from build123d import *

# Parameters (mm, degrees)
SKETCH1_W           = 226
SKETCH1_H           = 100
SKETCH1_W_2         = 30
SKETCH1_H_2         = 30
SKETCH1_W_3         = 5
SKETCH1_H_3         = 60
SKETCH1_H_4         = 5
SKETCH1_W_4         = 60
BOSS_EXTRUDE1_DEPTH = 5


with BuildPart() as part:
    # Sketch1 → Boss-Extrude1 (new body)
    # profile 1 of 9: a face of its own
    with BuildSketch(Plane(origin=(0, 0, 0), x_dir=(0, 0, -1), z_dir=(1, 0, 0))):
        Rectangle(SKETCH1_W, SKETCH1_H)
        with Locations((-88, 0)):
            Rectangle(SKETCH1_W_2, SKETCH1_H_2, mode=Mode.SUBTRACT)
    # profile 2 of 9: a face of its own
    with BuildSketch(Plane(origin=(0, 0, 0), x_dir=(0, 0, -1), z_dir=(1, 0, 0))):
        with Locations((115.5, 0)):
            Rectangle(SKETCH1_W_3, SKETCH1_H_3)
    # profile 3 of 9: a face of its own
    with BuildSketch(Plane(origin=(0, 0, 0), x_dir=(0, 0, -1), z_dir=(1, 0, 0))):
        with Locations((83, 52.5)):
            Rectangle(SKETCH1_W_2, SKETCH1_H_4)
    # profile 4 of 9: a face of its own
    with BuildSketch(Plane(origin=(0, 0, 0), x_dir=(0, 0, -1), z_dir=(1, 0, 0))):
        with Locations((0, 52.5)):
            Rectangle(SKETCH1_W_4, SKETCH1_H_4)
    # profile 5 of 9: a face of its own
    with BuildSketch(Plane(origin=(0, 0, 0), x_dir=(0, 0, -1), z_dir=(1, 0, 0))):
        with Locations((83, -52.5)):
            Rectangle(SKETCH1_W_2, SKETCH1_H_4)
    # profile 6 of 9: a face of its own
    with BuildSketch(Plane(origin=(0, 0, 0), x_dir=(0, 0, -1), z_dir=(1, 0, 0))):
        with Locations((0, -52.5)):
            Rectangle(SKETCH1_W_4, SKETCH1_H_4)
    # profile 7 of 9: a face of its own
    with BuildSketch(Plane(origin=(0, 0, 0), x_dir=(0, 0, -1), z_dir=(1, 0, 0))):
        with Locations((-83, -52.5)):
            Rectangle(SKETCH1_W_2, SKETCH1_H_4)
    # profile 8 of 9: a face of its own
    with BuildSketch(Plane(origin=(0, 0, 0), x_dir=(0, 0, -1), z_dir=(1, 0, 0))):
        with Locations((-115.5, 0)):
            Rectangle(SKETCH1_W_3, SKETCH1_H_3)
    # profile 9 of 9: a face of its own
    with BuildSketch(Plane(origin=(0, 0, 0), x_dir=(0, 0, -1), z_dir=(1, 0, 0))):
        with Locations((-83, 52.5)):
            Rectangle(SKETCH1_W_2, SKETCH1_H_4)
    extrude(amount=BOSS_EXTRUDE1_DEPTH)


solid = part.part
The model under review builds one solid part; all positions refer to its coordinate system, in mm. A direction names the side the tool comes from. Give positions to 0.01 mm unless a question says otherwise; leave off trailing zeros. Loops run counter-clockwise (first coordinate to the right, second up) from the corner with the lowest first, then second, coordinate; pieces in that order, holes last. Notation, with made-up numbers: (5, -10) -> (22, -10) arc R14 cw to (22, 17) -> close; hole circle Ø10 at (-7, -32). An arc over 180 degrees is marked (long way). Answer as a JSON object with one key per item and string values. Group by question number.
Q1. Insertion check: pin 1 (1.5 mm diameter, centred on x = 3.5, y = 52, fed in from -Z); pin 2 (1.5 mm diameter, centred on x = 2.5, z = 116, fed in from -Y); pin 3 (1.5 mm diameter, centred on x = 1.5, y = 51.5, fed in from +Z). Each pin has a flat end and moves straight along its axis. Give the tip position at first contact, or say it passes through.
Q2. Take a section at C-C (y = 33). Write out the cut boundary in (x, z), plus the area to 3 significant figures.
Q3. Wall thickness on line 1 along Z through (x, y) = (2.45, -11); line 2 along Z through (x, y) = (3.4, 50.5); line 3 along Y through (x, z) = (4.35, -107.5): over which ranges is each line inside the solid? List them lowest first.
Q4. Take a section at A-A (y = -5.5). Write out the cut boundary in (x, z).
Q5. Draft analysis for pull direction Y (two halves, no side actions). For faces 6 (the flat face through (2, 52, 68)), 7 (the flat face through (2, -15, 88)), 8 (the flat face through (2, 50, 49)), state which applies: pulls with the +Y half, pulls with the -Y half, needs draft (parallel to the pull), parting line crosses it, or undercut.
Q6. Take a section at B-B (z = -50). Write out the cut boundary in (x, y), plus the area to 3 significant figures.
Q7. Tool access review of faces 1 (the flat face through (2, -53, -98)), 2 (the flat face through (2, 30, 116)), 3 (the flat face through (2, 15, 88)), 4 (the flat face through (2, 52, -68)), 5 (the flat face through (2, 52, -98)): name each direction out of +Z, -Z, +X, -X, +Y, -Y from which nothing blocks a thin tool from reaching the whole face with its end or side.
Answer below:
{
 "1": {"pin 1": "stops at z = -98", "pin 2": "stops at y = -30", "pin 3": "stops at z = 98"},
 "2": {"outline": "(0, -113) -> (5, -113) -> (5, 113) -> (0, 113) -> close", "area": "1,130 mm2"},
 "3": {"line 1": "z = -118 to 73, 103 to 118", "line 2": "z = -98 to -68, -30 to 30, 68 to 98", "line 3": "y = -50 to 50"},
 "4": {"outline": "(0, -118) -> (5, -118) -> (5, 73) -> (0, 73) -> close; (0, 103) -> (5, 103) -> (5, 118) -> (0, 118) -> close"},
 "5": {"face 6": "needs draft", "face 7": "undercut", "face 8": "pulls with the +Y half"},
 "6": {"outline": "(0, -50) -> (5, -50) -> (5, 50) -> (0, 50) -> close", "area": "500 mm2"},
 "7": {"face 1": "-Z, +X, -X, -Y", "face 2": "+Z, +X, -X, +Y", "face 3": "+X, -X", "face 4": "+X, -X, +Y", "face 5": "-Z, +X, -X, +Y"}
}
